```python
from build123d import *

# Parameters (mm, degrees)
SKETCH_1_R      = 8.8985
EXTRUDE_1_DEPTH = 13
CHAMFER_1_SIZE  = 1.1015


with BuildPart() as part:
    # Эскиз1 → Бобышка-Вытянуть1 (new body)
    with BuildSketch(Plane.XY):
        Polygon((0, 16.165807537), (-14, 8.082903769), (-14, -8.082903769), (0, -16.165807537), (14, -8.082903769), (14, 8.082903769), align=None)
        Circle(SKETCH_1_R, mode=Mode.SUBTRACT)
    extrude(amount=-EXTRUDE_1_DEPTH)

    # Эскиз2 → Вырез-Повернуть1 (revolve, cut)
    with BuildSketch(Plane(origin=(0, 0, 0), x_dir=(0, 0, -1), z_dir=(1, 0, 0))):
        Polygon((0, 13.965807537), (5.773502692, 23.965807537), (0, 23.965807537), align=None)
        Polygon((13, 23.965807537), (13, 13.965807537), (7.226497308, 23.965807537), align=None)
    revolve(axis=Axis((0, 0, 0), (0, 0, 1)), mode=Mode.SUBTRACT)

    # Фаска1
    chamfer_1_edges = [part.edges().sort_by_distance(p)[0] for p in [
        (-8.8985, 0, -13),
        (-8.8985, 0, 0),
    ]]
    chamfer(chamfer_1_edges, length=CHAMFER_1_SIZE)


solid = part.part
```
Model file for the job. Use its own axes, mm. Give positions to 0.01 mm unless a question says otherwise; leave off trailing zeros. Write each loop counter-clockwise with the first axis right and the second up, starting at its lowest first coordinate (ties: lowest second). Pieces come first, ordered by that corner, then holes. Notation, with made-up numbers: M -35.75,59 L -6.75,59 A20 cw -6.75,86 Z; hole C 17,44 d1. An arc over 180 degrees is marked long. Use a Markdown table: item, result.
1) Pin check, flat tip, straight feed: pin 1 (3 mm diameter, centred on x = 5.5, z = -9, fed in from -Y). Stop position of the tip, or through.
Responses:
| item | result |
|---|---|
| pin 1 | stops at y = -13.86 |
2) Drill centre lines: line 1 (Y direction, x = 0, z = -8.25); line 2 (X direction, y = 3.5, z = -4.25); line 3 (X direction, y = -6, z = -10.75). Where is each one in solid material? Low to high. Write a range as from..to.
Responses:
| item | result |
|---|---|
| line 1 | y = -16.17..-8.9, 8.9..16.17 |
| line 2 | x = -14..-8.18, 8.18..14 |
| line 3 | x = -14..-6.57, 6.57..14 |
3) Cut at B-B (z = -2.5). List the corners of the cut face in (x, y), and give its area (3 significant figures).
Responses:
| item | result |
|---|---|
| outline | M -14,-8.08 L 0,-16.17 L 14,-8.08 L 14,8.08 L 0,16.17 L -14,8.08 Z; hole C 0,0 d17.8 |
| area | 430 mm2 |
4) Pull direction X, two halves, no side cores. Call faces 1 (the cylindrical face through (-1.929, -8.687, -6.424)), 2 (the flat face through (-10, 3, -13)), 3 (the flat face through (-14, 0, -6)), 4 (the flat face through (14, 0, -6)): +X half, -X half, draft (parallel to the pull), parting line (faces both ways), or undercut.
Responses:
| item | result |
|---|---|
| face 1 | undercut |
| face 2 | draft |
| face 3 | -X half |
| face 4 | +X half |
